```python
from build123d import *

# Parameters (mm, degrees)
SKETCH_1_R          = 17
SKETCH_1_R_2        = 14
EXTRUDE_1_DEPTH     = 15
SKETCH_2_R          = 15.1
SKETCH_2_R_2        = 14
CUT_EXTRUDE_1_DEPTH = 1.7
EXTRUDE_2_DEPTH     = 5
FILLET_1_R          = 1
FILLET_2_R          = 1


with BuildPart() as part:
    # 草图1 → 凸台-拉伸1 (new body)
    with BuildSketch(Plane(origin=(0, 0, 0), x_dir=(1, 0, 0), z_dir=(0, 1, 0))):
        Circle(SKETCH_1_R)
        Circle(SKETCH_1_R_2, mode=Mode.SUBTRACT)
    extrude(amount=EXTRUDE_1_DEPTH)

    # 草图2 → 切除-拉伸1 (cut)
    with BuildSketch(Plane(origin=(0, 0, 0), x_dir=(1, 0, 0), z_dir=(0, 1, 0))):
        Circle(SKETCH_2_R)
        Circle(SKETCH_2_R_2, mode=Mode.SUBTRACT)
    extrude(amount=CUT_EXTRUDE_1_DEPTH, mode=Mode.SUBTRACT)

    # 草图3 → 凸台-拉伸2 (add)
    with BuildSketch(Plane(origin=(0, 15, 0), x_dir=(1, 0, 0), z_dir=(0, 1, 0))):
        with BuildLine():
            Line((-22, 5), (-22, -5))
            Line((-22, -5), (-16.248076809, -5))
            ThreePointArc((-16.248076809, -5), (-17, 0), (-16.248076809, 5))
            Line((-16.248076809, 5), (-22, 5))
        make_face()
    extrude(amount=-EXTRUDE_2_DEPTH)

    # 草图11 → 旋转1 (revolve)
    with BuildSketch(Plane.XY):
        Polygon((13.5, 50), (14, 15), (16.933723731, 15), (15.5, 50), align=None)
    revolve(axis=Axis((0, 50, 0), (0, -1, 0)))

    # 圆角1
    fillet_1_edges = [part.edges().sort_by_distance(p)[0] for p in [
        (-17, 0, 0),
        (-15.5, 50, 0),
        (-13.5, 50, 0),
    ]]
    fillet(fillet_1_edges, radius=FILLET_1_R)

    # 圆角2
    fillet_2_edges = [part.edges().sort_by_distance(p)[0] for p in [
        (-16.248076809, 12.5, -5),
        (-16.248076809, 12.5, 5),
    ]]
    fillet(fillet_2_edges, radius=FILLET_2_R)


solid = part.part
```
Can you work these out from the model? Positions are in its coordinate system, mm. A direction names the side the tool comes from. Give positions to 0.01 mm unless a question says otherwise; leave off trailing zeros. Loops run counter-clockwise (first coordinate to the right, second up) from the corner with the lowest first, then second, coordinate; pieces in that order, holes last. Notation, with made-up numbers: M 43,-9.5 L 85,-9.5 A16 cw 85,-3.5 Z; hole C 19.5,18 d7. An arc over 180 degrees is marked long. One line per item, written item: value.
(1) Suppose I cut it at B-B on y = 38. List the corners of the cut face in (x, z) for me.
Returned:
outline: C 0,0 d31.98; hole C 0,0 d27.34
(2) Will these pins go through, and if not, where does the flat tip stop? pin 1 (10 mm diameter, centred on x = -8, z = -5, fed in from +Y); pin 2 (3 mm diameter, centred on y = 43.5, z = 11.5, fed in from +X); pin 3 (2 mm diameter, centred on y = 30.5, z = 6.5, fed in from +X).
Returned:
pin 1: y = 50
pin 2: x = 12.19
pin 3: x = 15.35
(3) We'd pull the mould along Z, two halves only. Please class faces 4 (the face through (12.932, 8.257, 5.362)), 5 (the face through (15.48, 32.26, 4.87)), 6 (the face through (-10, 0, 12)): released by +Z, released by -Z, zero draft, split by the parting line, or undercut.
Returned:
face 4: undercut
face 5: split by the parting line
face 6: zero draft
(4) Which directions (+Z, -Z, +X, -X, +Y, -Y) give clear straight access to the entire face, cutting with the end or side of a thin tool? Please do faces 1 (the face through (9, 1.7, 11)), 2 (the face through (-19, 13, -5)), 3 (the face through (-20, 13, 5)).
Returned:
face 1: -Y
face 2: -Z, -X, +Y, -Y
face 3: +Z, -X, +Y, -Y
(5) I need wall thicknesses on line 1 (Z direction, x = 0, y = 8); line 2 (Z direction, x = 0, y = 1.35). Which ranges of each line are inside material? Lowest first, please.
Returned:
line 1: -17 to -14, 14 to 17
line 2: -17 to -15.1, 15.1 to 17
(6) Suppose I cut it at A-A on y = 18.5. List the corners of the cut face in (x, z) for me, plus the area to 3 significant figures.
Returned:
outline: C 0,0 d33.58; hole C 0,0 d27.9
area: 274 mm^2
